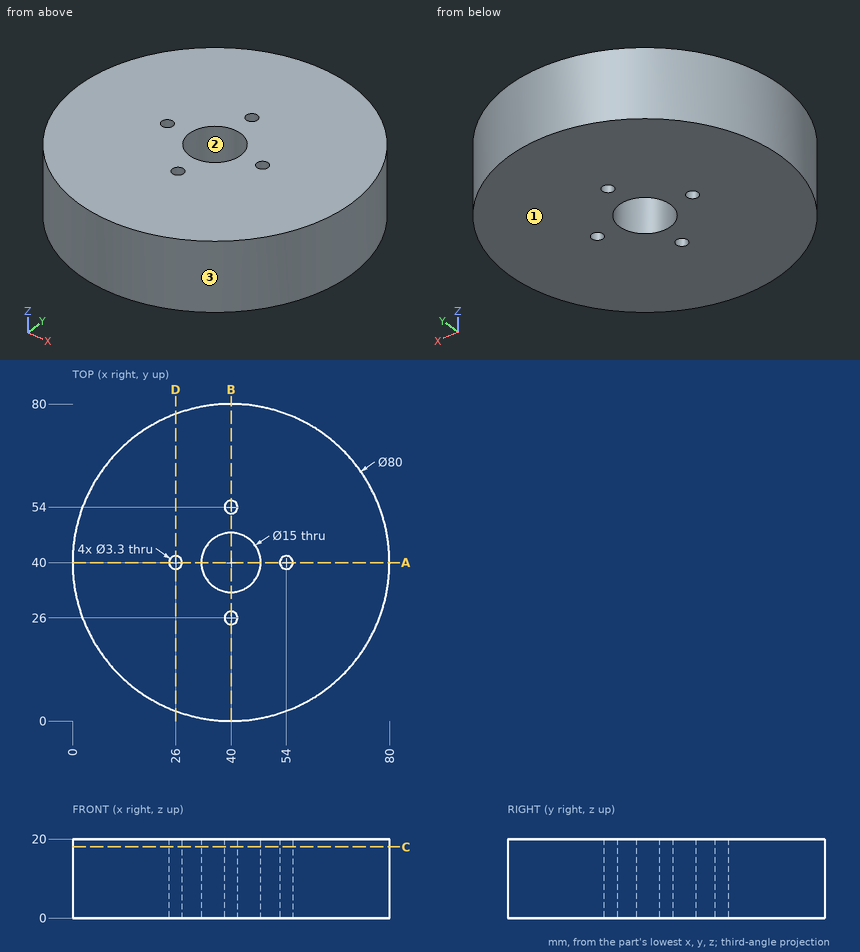
Here's the drawing with two shaded views (mm, measured from the low corner). I have some questions. Coordinates: 2 decimals unless noted, no trailing zeros. Order: outer loops, then holes, each group sorted by start corner. A loop starts at its lowest first (then second) coordinate and runs counter-clockwise, first axis right, second up.
Item 1: If we section it at A-A on y = 40: List the corners of the cut face in (x, z) for me.
Result sheet:
outline: (0, 0) - (24.35, 0) - (24.35, 20) - (0, 20) - close; (27.65, 0) - (32.5, 0) - (32.5, 20) - (27.65, 20) - close; (47.5, 0) - (52.35, 0) - (52.35, 20) - (47.5, 20) - close; (55.65, 0) - (80, 0) - (80, 20) - (55.65, 20) - close
Item 2: If we mould it in two halves opening along Y, with no side actions, what happens to the marked faces 1, 2 and 3? For each: +Y half, -Y half, draft (parallel to the pull), parting line (faces both ways), or undercut.
Result sheet:
face 1: draft
face 2: undercut
face 3: parting line
Item 3: If we section it at C-C on z = 18: List the corners of the cut face in (x, y) for me.
Result sheet:
outline: circle Ø80 at (40, 40); hole circle Ø3.3 at (26, 40); hole circle Ø15 at (40, 40); hole circle Ø3.3 at (40, 26); hole circle Ø3.3 at (40, 54); hole circle Ø3.3 at (54, 40)
Item 4: If we section it at D-D on x = 26: List the corners of the cut face in (y, z) for me, plus the area to 3 significant figures.
Result sheet:
outline: (2.53, 0) - (38.35, 0) - (38.35, 20) - (2.53, 20) - close; (41.65, 0) - (77.47, 0) - (77.47, 20) - (41.65, 20) - close
area: 1,430 mm2
Item 5: For P1, Ø4, axis at x = 21, z = 3, coming from the -Y side; P2, Ø8, axis at x = 52.5, z = 2.5, coming from the +Y side; P3, Ø3, axis at y = 53.5, z = 4, coming from the +X side, each with a flat end and sliding along its axis, tell me the tip position at first contact or that it passes through.
Result sheet:
P1: stops at y = 3.79
P2: stops at y = 79.09
P3: stops at x = 78.16
Item 6: I need wall thicknesses on line 1 (Y direction, x = 40, z = 11.25); line 2 (Y direction, x = 26, z = 15.5); line 3 (Y direction, x = 53, z = 4). Which ranges of each line are inside material? Lowest first, please.
Result sheet:
line 1: y = 0 to 24.35, 27.65 to 32.5, 47.5 to 52.35, 55.65 to 80
line 2: y = 2.53 to 38.35, 41.65 to 77.47
line 3: y = 2.17 to 38.69, 41.31 to 77.83
